```python
from build123d import *

# Parameters (mm, degrees)
SKETCH1_W           = 85
SKETCH1_H           = 56
BOSS_EXTRUDE1_DEPTH = 1.5
FILLET1_R           = 2.5
SKETCH2_R           = 1.3
CUT_EXTRUDE1_DEPTH  = 51.916598472
SKETCH3_W           = 14
SKETCH3_H           = 14
BOSS_EXTRUDE2_DEPTH = 0.1
SKETCH4_W           = 50.5
SKETCH4_H           = 5.2
BOSS_EXTRUDE3_DEPTH = 22
SKETCH5_W           = 7.5
SKETCH5_H           = 5.5
BOSS_EXTRUDE4_DEPTH = 3
SKETCH6_W           = 4
SKETCH6_H           = 22.4
SKETCH6_W_2         = 15
SKETCH6_H_2         = 11.5
SKETCH6_W_3         = 7.4
SKETCH6_H_3         = 15
BOSS_EXTRUDE5_DEPTH = 6
SKETCH7_W           = 21.5
SKETCH7_H           = 15.9
BOSS_EXTRUDE6_DEPTH = 13.5
SKETCH7_3_W         = 17
SKETCH7_3_H         = 15.4
BOSS_EXTRUDE7_DEPTH = 16


with BuildPart() as part:
    # Sketch1 → Boss-Extrude1 (new body)
    with BuildSketch(Plane(origin=(0, 0, 0), x_dir=(1, 0, 0), z_dir=(0, 1, 0))):
        Rectangle(SKETCH1_W, SKETCH1_H)
    extrude(amount=BOSS_EXTRUDE1_DEPTH)

    # Fillet1
    fillet1_edges = [part.edges().sort_by_distance(p)[0] for p in [
        (42.5, 0.75, 28),
        (-42.5, 0.75, 28),
        (-42.5, 0.75, -28),
        (42.5, 0.75, -28),
    ]]
    fillet(fillet1_edges, radius=FILLET1_R)

    # Sketch2 → Cut-Extrude1 (cut, through all)
    with BuildSketch(Plane(origin=(0, 1.5, 0), x_dir=(1, 0, 0), z_dir=(0, 1, 0))):
        with Locations(Location((-38.95, -24.45, 0), (0, 0, 270))):
            Circle(SKETCH2_R)
        with Locations(Location((-38.95, 24.45, 0), (0, 0, 270))):
            Circle(SKETCH2_R)
        with Locations(Location((18.95, 24.45, 0), (0, 0, 270))):
            Circle(SKETCH2_R)
        with Locations(Location((18.95, -24.45, 0), (0, 0, 270))):
            Circle(SKETCH2_R)
    extrude(amount=-CUT_EXTRUDE1_DEPTH, mode=Mode.SUBTRACT)

    # Sketch3 → Boss-Extrude2 (add)
    with BuildSketch(Plane(origin=(0, 1.5, 0), x_dir=(1, 0, 0), z_dir=(0, 1, 0))):
        with Locations((-15.5, 4)):
            Rectangle(SKETCH3_W, SKETCH3_H)
    extrude(amount=BOSS_EXTRUDE2_DEPTH)

    # Sketch4 → Boss-Extrude3 (add)
    with BuildSketch(Plane(origin=(0, 1.5, 0), x_dir=(1, 0, 0), z_dir=(0, 1, 0))):
        with Locations((-9.75, 23.9)):
            Rectangle(SKETCH4_W, SKETCH4_H)
    extrude(amount=BOSS_EXTRUDE3_DEPTH)

    # Sketch5 → Boss-Extrude4 (add)
    with BuildSketch(Plane(origin=(0, 1.5, 0), x_dir=(1, 0, 0), z_dir=(0, 1, 0))):
        with Locations((-32.25, -26.25)):
            Rectangle(SKETCH5_W, SKETCH5_H)
    extrude(amount=BOSS_EXTRUDE4_DEPTH)

    # Sketch6 → Boss-Extrude5 (add)
    with BuildSketch(Plane(origin=(0, 1.5, 0), x_dir=(1, 0, 0), z_dir=(0, 1, 0))):
        with Locations((2, -16.8)):
            Rectangle(SKETCH6_W, SKETCH6_H)
        with Locations((-39.5, 0.2)):
            Rectangle(SKETCH6_W, SKETCH6_H)
        with Locations((-11.5, -23.25)):
            Rectangle(SKETCH6_W_2, SKETCH6_H_2)
        with Locations((9.7, -23)):
            Rectangle(SKETCH6_W_3, SKETCH6_H_3)
    extrude(amount=BOSS_EXTRUDE5_DEPTH)

    # Sketch7 → Boss-Extrude6 (add)
    with BuildSketch(Plane(origin=(0, 1.5, 0), x_dir=(1, 0, 0), z_dir=(0, 1, 0))):
        with Locations((33.75, -18.05)):
            Rectangle(SKETCH7_W, SKETCH7_H)
    extrude(amount=BOSS_EXTRUDE6_DEPTH)

    # Sketch7_3 → Boss-Extrude7 (add)
    with BuildSketch(Plane(origin=(0, 1.5, 0), x_dir=(1, 0, 0), z_dir=(0, 1, 0))):
        with Locations((36, 18.8)):
            Rectangle(SKETCH7_3_W, SKETCH7_3_H)
        with Locations((36, 0.8)):
            Rectangle(SKETCH7_3_W, SKETCH7_3_H)
    extrude(amount=BOSS_EXTRUDE7_DEPTH)


solid = part.part
```
Can you work these out from the model? Positions are in its coordinate system, mm. A direction names the side the tool comes from. Round coordinates to 2 decimals unless told otherwise and drop trailing zeros. Loops run counter-clockwise (first coordinate to the right, second up) from the corner with the lowest first, then second, coordinate; pieces in that order, holes last.
Item 1: Will these pins go through, and if not, where does the flat tip stop? pin 1 Ø0.9 at (x, y) = (-33.5, 3) entering from +Z; pin 2 Ø2 at (x, y) = (1, 4.5) entering from -Z; pin 3 Ø15.5 at (x, z) = (-16, -3) entering from +Y.
Item 2: If we mould it in two halves opening along Z, with no side actions, what happens to faces 1 (the flat face through (-32, 3, 23.5)), 2 (the flat face through (-10, 12, -26.5)), 3 (the flat face through (-40, 4, 11)), 4 (the flat face through (-19, 4, 23))? For each: +Z half, -Z half, draft (parallel to the pull), parting line (faces both ways), or undercut.
Item 3: Suppose I cut it at D-D, the plane z = -18.5. Write out the boundary of the cut face in (x, y), then the cut area to 4 significant figures.
Item 4: Suppose I cut it at C-C, the plane x = 18.95. Write out the boundary of the cut face in (y, z).
Item 5: Suppose I cut it at B-B, the plane y = 10.5. Write out the boundary of the cut face in (x, z).
Item 6: Which directions (+Z, -Z, +X, -X, +Y, -Y) give clear straight access to the entire face, cutting with the end or side of a thin tool? Please do faces 5 (the flat face through (36, 9, 6.9)), 6 (the flat face through (-10, 12, -21.3)), 7 (the flat face through (-41.5, 4, 0)), 8 (the flat face through (23, 8, 18)), 9 (the flat face through (13.4, 4, 23)).
Item 7: Please list where these lines run through material, in increasing order: L1, parallel to X at y = 0.9, z = -24.45; L2, parallel to X at y = 5, z = 17; L3, parallel to Z at x = 39, y = 11.
Item 8: Suppose I cut it at A-A, the plane z = 24.45. State how many separate pieces and enclosed holes the cut face has, then the cut area to 3 significant figures.
Reported:
1. pin 1: stops at z = 29
1. pin 2: stops at z = -26.5
1. pin 3: stops at y = 1.6
2. face 1: undercut
2. face 2: -Z half
2. face 3: +Z half
2. face 4: draft
3. outline: (-42.5, 0) - (42.5, 0) - (42.5, 1.5) - (44.5, 1.5) - (44.5, 17.5) - (27.5, 17.5) - (27.5, 1.5) - (-42.5, 1.5) - close
3. area: 399.5 mm2
4. outline: (0, -28) - (1.5, -28) - (1.5, -25.75) - (0, -25.75) - close; (0, -23.15) - (1.5, -23.15) - (1.5, 23.15) - (0, 23.15) - close; (0, 25.75) - (1.5, 25.75) - (1.5, 28) - (0, 28) - close
5. outline: (-35, -26.5) - (15.5, -26.5) - (15.5, -21.3) - (-35, -21.3) - close; (23, 10.1) - (44.5, 10.1) - (44.5, 26) - (23, 26) - close; (27.5, -26.5) - (44.5, -26.5) - (44.5, -11.1) - (27.5, -11.1) - close; (27.5, -8.5) - (44.5, -8.5) - (44.5, 6.9) - (27.5, 6.9) - close
6. face 5: +X, +Y
6. face 6: -X, +Y
6. face 7: +Z, -Z, -X, +Y
6. face 8: +Z, -Z, +Y
6. face 9: +Z, +Y
7. L1: x = -42.5 to -40.25, -37.65 to 17.65, 20.25 to 42.5
7. L2: x = 0 to 4, 6 to 13.4, 23 to 44.5
7. L3: z = -26.5 to -11.1, -8.5 to 6.9, 10.1 to 26
8. separate pieces: 3
8. enclosed holes: 0
8. area: 591 mm2
